```python
from build123d import *

# Parameters (mm, degrees)
SKETCH2_R           = 4.7625
BOSS_EXTRUDE1_DEPTH = 8.89
CUT_EXTRUDE1_DEPTH  = 3.175


with BuildPart() as part:
    # Sketch1 → Revolve1 (revolve)
    with BuildSketch(Plane.XY):
        with BuildLine():
            Line((0, 0), (-3.175, 0))
            Line((-3.175, 0), (-3.175, 12.7))
            add(Edge.make_bspline(
                [(-3.175, 12.7), (-3.175, 19.05), (0, 6.35), (3.175, 19.05), (3.175, 12.7)],
                knots=[0, 0, 0, 0, 0, 1, 1, 1, 1, 1], degree=4))
            Line((3.175, 12.7), (3.175, 0))
            Line((3.175, 0), (0, 0))
        make_face()
    revolve(axis=Axis((0, 0, 0), (-1, 0, 0)))

    # Sketch2 → Boss-Extrude1 (add)
    with BuildSketch(Plane(origin=(3.175, 0, 0), x_dir=(0, 0, -1), z_dir=(1, 0, 0))):
        Circle(SKETCH2_R)
        with BuildLine():
            Line((1.132738197, -2.273434446), (2.250324949, 1.177980315))
            ThreePointArc((2.250324949, 1.177980315), (0.782467236, 2.416473676), (-1.132738197, 2.273434446))
            Line((-1.132738197, 2.273434446), (-2.250324949, -1.177980315))
            ThreePointArc((-2.250324949, -1.177980315), (-0.782467236, -2.416473676), (1.132738197, -2.273434446))
        make_face(mode=Mode.SUBTRACT)
    extrude(amount=BOSS_EXTRUDE1_DEPTH)

    # Sketch2_2 → Cut-Extrude1 (cut)
    with BuildSketch(Plane(origin=(3.175, 0, 0), x_dir=(0, 0, -1), z_dir=(1, 0, 0))):
        with BuildLine():
            Line((1.132738197, -2.273434446), (2.250324949, 1.177980315))
            ThreePointArc((2.250324949, 1.177980315), (0.782467236, 2.416473676), (-1.132738197, 2.273434446))
            Line((-1.132738197, 2.273434446), (-2.250324949, -1.177980315))
            ThreePointArc((-2.250324949, -1.177980315), (-0.782467236, -2.416473676), (1.132738197, -2.273434446))
        make_face()
    extrude(amount=-CUT_EXTRUDE1_DEPTH, mode=Mode.SUBTRACT)


solid = part.part
```
Here's how the part is built. I have some questions about the finished solid (model axes, mm). A direction names the side the tool comes from. Give positions to 0.01 mm unless a question says otherwise; leave off trailing zeros. Order: outer loops, then holes, each group sorted by start corner. A loop starts at its lowest first (then second) coordinate and runs counter-clockwise, first axis right, second up. Notation, with made-up numbers: (-24.75, 12) - (7.25, 12) arc R16 cw to (7.25, 27) - close; hole circle Ø1 at (-18, 62.5). An arc over 180 degrees is marked (long way). Answer as a JSON object with one key per item and string values. Group by question number.
Item 1: Please list where these lines run through material, in increasing order: probe 1 along X at (y, z) = (-10.25, 0) (3 decimals); probe 2 along Z at (x, y) = (-0.25, -11); probe 3 along Y at (x, z) = (0.75, -2.75).
Item 2: If we section it at A-A on x = 5.5: Please give me the cut outline in (y, z) (1 decimal), and give its area (3 significant figures).
Item 3: For P1, Ø5, axis at y = -0.5, z = 0.5, coming from the +X side (3 decimals); P2, Ø4, axis at y = 4.5, z = 5.5, coming from the +X side (3 decimals); P3, Ø2, axis at x = 9.5, y = -3.5, coming from the +Z side; P4, Ø1, axis at x = 10, y = -7, coming from the -Z side, each with a flat end and sliding along its axis, tell me the tip position at first contact or that it passes through.
Item 4: Which directions (+Z, -Z, +X, -X, +Y, -Y) give clear straight access to the entire face, cutting with the end or side of a thin tool? Please do faces 1 (the cylindrical face through (5.948, -2.408, 0.809)), 2 (the flat face through (-3.175, 0, 0)).
Result set:
{
 "1": {"probe 1": "-3.175 to 3.175", "probe 2": "-7.84 to 7.84", "probe 3": "-13.33 to 13.33"},
 "2": {"outline": "circle Ø9.5 at (0, 0); hole (-2.3, -1.1) - (1.2, -2.3) arc R2.5 ccw to (2.3, 1.1) - (-1.2, 2.3) arc R2.5 ccw to start", "area": "54.8 mm²"},
 "3": {"P1": "x = 12.065", "P2": "x = 3.175", "P3": "z = 4.05", "P4": "through"},
 "4": {"face 1": "+X", "face 2": "+Z, -Z, -X, +Y, -Y"}
}
